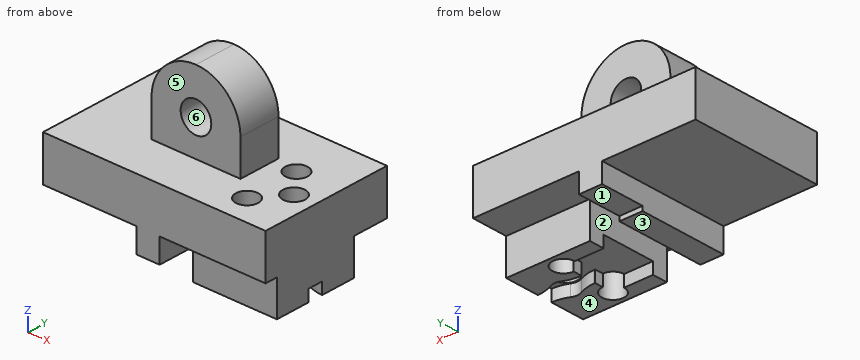
```python
from build123d import *

# Parameters (mm, degrees)
F0_W      = 31.75
F0_H      = 6.35
F1_DEPTH  = 19.05
F2_W      = 12.7
F2_H      = 5.969
F3_DEPTH  = 11.43
F4_R      = 6.34999
F5_R      = 2.1844
F6_DEPTH  = 25.4
F7_W      = 11.938
F7_H      = 12.065
F8_DEPTH  = 5.08
F9_W      = 5.715
F9_H      = 7.747
F10_DEPTH = 1.651
F11_R     = 1.5875
F12_DEPTH = 25.4
F13_W     = 3.302
F13_H     = 19.05
F14_DEPTH = 3.429
F15_W     = 3.302
F15_H     = 6.35
F16_DEPTH = 0.635
F18_DEPTH = 1.651
F19_R     = 5.08


# Not quite as in the source:
# - a fillet or chamfer is up to 0.001 mm smaller than in the source, because OpenCascade refuses the exact size


with BuildPart() as f1:
    # F0 (on Front) → F1 (new body)
    with BuildSketch(Plane.XZ):
        Rectangle(F0_W, F0_H)
    extrude(amount=F1_DEPTH)

    # F2 (on face) → F3 (join)
    with BuildSketch(Plane.XY.offset(3.175)):
        with Locations((0, -9.525)):
            Rectangle(F2_W, F2_H)
    extrude(amount=F3_DEPTH)

    # F4 (radius 6.35 in the source; OpenCascade refuses exactly that, so slightly less here)
    f4_edges = [f1.edges().sort_by_distance(p)[0] for p in [
        (-6.35, -9.525, 14.605),
        (6.35, -9.525, 14.605),
    ]]
    fillet(f4_edges, radius=F4_R)

    # F5 (on face) → F6 (cut)
    with BuildSketch(Plane.XZ.offset(12.5095)):
        with Locations((0, 8.255)):
            Circle(F5_R)
    extrude(amount=-F6_DEPTH, mode=Mode.SUBTRACT)

    # F7 (on face) → F8 (join)
    with BuildSketch(Plane(origin=(0, 0, -3.175), x_dir=(1, 0, 0), z_dir=(0, 0, -1))):
        with Locations((9.906, 11.2395)):
            Rectangle(F7_W, F7_H)
    extrude(amount=F8_DEPTH)

    # F9 (on face) → F10 (cut)
    with BuildSketch(Plane(origin=(0, 0, -8.255), x_dir=(1, 0, 0), z_dir=(0, 0, -1))):
        with Locations((6.7945, 11.2395)):
            Rectangle(F9_W, F9_H)
    extrude(amount=-F10_DEPTH, mode=Mode.SUBTRACT)

    # F11 (on face) → F12 (cut)
    with BuildSketch(Plane(origin=(0, 0, -8.255), x_dir=(1, 0, 0), z_dir=(0, 0, -1))):
        with Locations((9.652, 15.113)):
            Circle(F11_R)
        with Locations((9.652, 7.366)):
            Circle(F11_R)
        with Locations((12.827, 11.2395)):
            Circle(F11_R)
    extrude(amount=-F12_DEPTH, mode=Mode.SUBTRACT)

    # F13 (on face) → F14 (join)
    with BuildSketch(Plane(origin=(0, 0, -3.175), x_dir=(1, 0, 0), z_dir=(0, 0, -1))):
        with Locations((-0.889, 9.525)):
            Rectangle(F13_W, F13_H)
    extrude(amount=F14_DEPTH)

    # F15 (on face) → F16 (cut)
    with BuildSketch(Plane(origin=(0, 0, -6.604), x_dir=(1, 0, 0), z_dir=(0, 0, -1))):
        with Locations((-0.889, 3.175)):
            Rectangle(F15_W, F15_H)
    extrude(amount=-F16_DEPTH, mode=Mode.SUBTRACT)

    # F17 (on face) → F18 (cut)
    with BuildSketch(Plane(origin=(0, 0, -8.255), x_dir=(1, 0, 0), z_dir=(0, 0, -1))):
        with BuildLine():
            Line((11.4142141882, 12.319), (9.652, 12.319))
            Line((9.652, 12.319), (9.652, 10.16))
            Line((9.652, 10.16), (11.4142141882, 10.16))
            ThreePointArc((11.4142141882, 10.16), (12.827, 9.4615), (14.2397858118, 10.16))
            Line((14.2397858118, 10.16), (15.875, 10.16))
            Line((15.875, 10.16), (15.875, 12.319))
            Line((15.875, 12.319), (14.2397858118, 12.319))
            ThreePointArc((14.2397858118, 12.319), (12.827, 13.0175), (11.4142141882, 12.319))
        make_face()
    extrude(amount=-F18_DEPTH, mode=Mode.SUBTRACT)

    # F19
    f19_edges = [f1.edges().sort_by_distance(p)[0] for p in [
        (11.414214, -12.319, -7.4295),
        (14.239786, -12.319, -7.4295),
        (11.414214, -10.16, -7.4295),
        (14.239786, -10.16, -7.4295),
    ]]
    fillet(f19_edges, radius=F19_R)


solid = f1.part
```
Source: CAD feature listing. Evaluate the final solid. Frame: model axes, mm. Face numbers are marked on the shaded views. A direction names the side the tool comes from. Round coordinates to 2 decimals unless told otherwise and drop trailing zeros. Loops run counter-clockwise (first coordinate to the right, second up) from the corner with the lowest first, then second, coordinate; pieces in that order, holes last.
(1) Section query A-A (z = -4.25). Give the number of separate pieces and of enclosed holes in the cut face, and give its area (3 significant figures).
From the geometry:
separate pieces: 2
enclosed holes: 3
area: 183 mm2
(2) Material intervals for probe 1 along X at (y, z) = (-7.25, -5.75) (3 decimals); probe 2 along X at (y, z) = (-8, -4.5) (3 decimals); probe 3 along X at (y, z) = (-5.25, -4.5) (3 decimals), sorted ascending.
From the geometry:
probe 1: x = -2.54 to 0.762, 3.937 to 8.069, 11.235 to 15.875
probe 2: x = -2.54 to 0.762, 3.937 to 8.197, 11.107 to 15.875
probe 3: x = -2.54 to 0.762, 3.937 to 15.875
(3) Pull-direction query (Z, two-part tool) for the marked faces 4, 5 and 6; classes: +Z half, -Z half, draft (parallel to the pull), parting line (faces both ways), or undercut.
From the geometry:
face 4: -Z half
face 5: draft
face 6: undercut
(4) Section query D-D (z = 7). Output: boundary loops of the cut face in (x, y), and give its area (3 significant figures).
From the geometry:
outline: (-6.35, -12.51) - (-1.79, -12.51) - (-1.79, -6.54) - (-6.35, -6.54) - close; (1.79, -12.51) - (6.35, -12.51) - (6.35, -6.54) - (1.79, -6.54) - close
area: 54.5 mm2
(5) Access query for the marked faces 1, 2 and 3. Directions: +Z, -Z, +X, -X, +Y, -Y. A direction counts if a zero-diameter tool reaches every point of the face in a straight line with its end or side. Return the directions, or none.
From the geometry:
face 1: -Z, -X, +Y
face 2: -Z, +Y, -Y
face 3: -Z, -X, +Y, -Y
(6) Contact query for flat-ended pins moving along their axis: pin 1 Ø10 at (x, y) = (-1, -7.5) entering from +Z (3 decimals); pin 2 Ø4 at (x, y) = (9.652, -15.113) entering from +Z (3 decimals); pin 3 Ø1 at (y, z) = (-16, -5) entering from -X; pin 4 Ø4 at (y, z) = (-8, 7.5) entering from +X. Output: stop coordinate, or through.
From the geometry:
pin 1: stops at z = 14.605
pin 2: stops at z = 3.175
pin 3: stops at x = -2.54
pin 4: stops at x = 6.35
(7) Section query B-B (y = -14.5). Output: boundary loops of the cut face in (x, z) (3 decimals).
From the geometry:
outline: (-15.875, -3.175) - (-2.54, -3.175) - (-2.54, -6.604) - (0.762, -6.604) - (0.762, -3.175) - (3.937, -3.175) - (3.937, -6.604) - (8.188, -6.604) - (8.188, 3.175) - (-15.875, 3.175) - close; (11.116, -8.255) - (15.875, -8.255) - (15.875, 3.175) - (11.116, 3.175) - close
